Check sheet for the modelled part. Datum: model origin and axes. Units: mm. A direction names the side the tool comes from. Give positions to 0.01 mm unless a question says otherwise; leave off trailing zeros. Order: outer loops, then holes, each group sorted by start corner. A loop starts at its lowest first (then second) coordinate and runs counter-clockwise, first axis right, second up.
Item 1: Sectioned sample at B-B on x = 7. Record the boundary of the cut face in (y, z), and give its area (3 significant figures).
Item 2: Gauge pin test, flat ends, axial feed: P1, Ø2.5, axis at y = -3.5, z = -4.5, coming from the -X side; P2, Ø1, axis at y = 6, z = 1, coming from the +X side; P3, Ø3, axis at x = 22.5, z = 1.5, coming from the +Y side. Record the tip position at first contact, or that the pin passes through.
Item 3: Release check for a two-part mould opening along Z. For faces 5 (the conical face through (23.8, 5.1, -3)), 6 (the flat face through (1.972, -2.898, 4.927)), 7 (the flat face through (-6, 0, 0)) record: released by +Z, released by -Z, zero draft, split by the parting line, or undercut.
Item 4: Sectioned sample at A-A on x = 0.5. Record the boundary of the cut face in (y, z).
Item 5: Access from +Z, -Z, +X, -X, +Y, -Y to the whole of each face (thin tool, end or side, straight path). Record for faces 1 (the flat face through (18, 6, 0)), 2 (the flat face through (2, -5.716, 0)), 3 (the flat face through (18, -3.1, 5.3)), 4 (the flat face through (21.042, -2.898, -4.927)).
Item 6: Material ranges on line 1 along X through (y, z) = (-4.25, 3.25); line 2 along X through (y, z) = (2.5, 5.75); line 3 along Y through (x, z) = (12.5, 0.25), recorded low to high.
from build123d import *

# Parameters (mm, degrees)
SKETCH2_OUTSIDE_W  = 23.168
SKETCH2_OUTSIDE_H  = 23.168
CUT_EXTRUDE1_DEPTH = 6
SKETCH3_OUTSIDE_W  = 23.168
SKETCH3_OUTSIDE_H  = 23.168
CUT_EXTRUDE2_DEPTH = 4
CHAMFER1_SIZE      = 0.5


with BuildPart() as part:
    # Sketch1 → Revolve1 (revolve)
    with BuildSketch(Plane(origin=(0, 0, 0), x_dir=(1, 0, 0), z_dir=(0, 1, 0))):
        Polygon((0, 6.6), (0, 3), (-6, 3), (-6, 0), (29.2, 0), (29.2, 2.4), (24, 2.4), (24, 6.6), align=None)
    revolve(axis=Axis((-26.186440678, 0, 0), (1, 0, 0)))

    # Sketch2 outside → Cut-Extrude1 (cut)
    with BuildSketch(Plane(origin=(24, 0, 0), x_dir=(0, 0, -1), z_dir=(1, 0, 0))):
        Rectangle(SKETCH2_OUTSIDE_W, SKETCH2_OUTSIDE_H)
        Polygon((3.3, -5.715767665), (6.6, 0), (3.3, 5.715767665), (-3.3, 5.715767665), (-6.6, 0), (-3.3, -5.715767665), align=None, mode=Mode.SUBTRACT)
    extrude(amount=-CUT_EXTRUDE1_DEPTH, mode=Mode.SUBTRACT)

    # Sketch3 outside → Cut-Extrude2 (cut)
    with BuildSketch(Plane.ZY):
        Rectangle(SKETCH3_OUTSIDE_W, SKETCH3_OUTSIDE_H)
        Polygon((3.3, -5.715767665), (6.6, 0), (3.3, 5.715767665), (-3.3, 5.715767665), (-6.6, 0), (-3.3, -5.715767665), align=None, mode=Mode.SUBTRACT)
    extrude(amount=-CUT_EXTRUDE2_DEPTH, mode=Mode.SUBTRACT)

    # Sketch4 → Cut-Revolve1 (revolve, cut)
    with BuildSketch(Plane.XY):
        Polygon((22.019646918, 7.696120747), (25.980353082, 3.735414583), (25.980353082, 7.696120747), align=None)
    revolve(axis=Axis((-26.186440678, 0, 0), (1, 0, 0)), mode=Mode.SUBTRACT)

    # Chamfer1
    chamfer1_edges = [part.edges().sort_by_distance(p)[0] for p in [
        (24, 0, 2.4),
        (-6, 0, 3),
    ]]
    chamfer(chamfer1_edges, length=CHAMFER1_SIZE)


solid = part.part
Report:
1. outline: circle Ø13.2 at (0, 0)
1. area: 137 mm2
2. P1: stops at x = 0
2. P2: stops at x = 24
2. P3: stops at y = 5.72
3. face 5: released by -Z
3. face 6: released by +Z
3. face 7: zero draft
4. outline: (-5.72, -3.3) - (0, -6.6) - (5.72, -3.3) - (5.72, 3.3) - (0, 6.6) - (-5.72, 3.3) - close
5. face 1: +Z, -Z, +X, +Y
5. face 2: +Z, -Z, -X, -Y
5. face 3: +Z, +X, -Y
5. face 4: -Z, +X, -Y
6. line 1: x = 0 to 24
6. line 2: x = 4 to 18
6. line 3: y = -6.6 to 6.6
